from build123d import *

# Parameters (mm, degrees)
SCHIZZO1_W                   = 25
SCHIZZO1_H                   = 2
ESTRUSIONE_ESTRUSIONE1_DEPTH = 47
SCHIZZO2_W                   = 25
SCHIZZO2_H                   = 2
ESTRUSIONE_ESTRUSIONE2_DEPTH = 6
FORO_FILETTATO_M3X0_5_1_D    = 2.5
RACCORDO1_R                  = 5
ESTRUSIONE_ESTRUSIONE3_DEPTH = 4


with BuildPart() as part:
    # Schizzo1 → Estrusione-Estrusione1 (new body)
    with BuildSketch(Plane.XY):
        with Locations((-25, 9)):
            Rectangle(SCHIZZO1_W, SCHIZZO1_H)
    extrude(amount=-ESTRUSIONE_ESTRUSIONE1_DEPTH)

    # Schizzo2 → Estrusione-Estrusione2 (add)
    with BuildSketch(Plane.XY):
        with Locations((-25, 9)):
            Rectangle(SCHIZZO2_W, SCHIZZO2_H)
    extrude(amount=ESTRUSIONE_ESTRUSIONE2_DEPTH)

    # Foro filettato M3x0.5-1 (through all)
    with Locations(Plane(origin=(0, 10, 0), x_dir=(1, 0, 0), z_dir=(0, 1, 0))):
        with Locations((-25, -3)):
            Hole(FORO_FILETTATO_M3X0_5_1_D / 2)

    # Raccordo1
    raccordo1_edges = [part.edges().sort_by_distance(p)[0] for p in [
        (-37.5, 9, 6),
        (-12.5, 9, 6),
    ]]
    fillet(raccordo1_edges, radius=RACCORDO1_R)

    # Schizzo5 → Estrusione-Estrusione3 (add)
    with BuildSketch(Plane(origin=(0, 0, -47), x_dir=(-1, 0, 0), z_dir=(0, 0, -1))):
        Polygon((12.5, 10), (12.5, 12), (37.5, 12), (37.5, 10), (37.5, 8), (12.5, 8), align=None)
    extrude(amount=ESTRUSIONE_ESTRUSIONE3_DEPTH)


solid = part.part
Design review of the part built by this model. Coordinates are the model's own, in mm. A direction names the side the tool comes from. Coordinates: 2 decimals unless noted, no trailing zeros. Write each loop counter-clockwise with the first axis right and the second up, starting at its lowest first coordinate (ties: lowest second). Pieces come first, ordered by that corner, then holes. Notation, with made-up numbers: (-26.75, 21.5) - (-17.75, 21.5) arc R9 ccw to (-17.75, 34.5) - close; hole circle Ø3 at (-32.5, -11). An arc over 180 degrees is marked (long way). Use one line per item in the form item = value.
Q1. The part is to be moulded in two halves that separate along Z. For faces 3 (the flat face through (-25, 10, -51)), 4 (the cylindrical face through (-26.155, 8.986, 3.479)), 5 (the flat face through (-25, 11, -47)), 6 (the flat face through (-12.5, 9, -25)), say which applies: +Z half, -Z half, draft (parallel to the pull), parting line (faces both ways), or undercut.
Taken from the geometry:
face_3 = -Z half
face_4 = undercut
face_5 = +Z half
face_6 = draft
Q2. Consider section D-D (y = 10.7). Write out the cut boundary in (x, z), plus the area to 3 significant figures.
Taken from the geometry:
outline = (-37.5, -51) - (-12.5, -51) - (-12.5, -47) - (-37.5, -47) - close
area = 100 mm^2
Q3. Insertion check: pin 1 Ø1.5 at (x, z) = (-25, 3) entering from +Y; pin 2 Ø1.5 at (x, z) = (-29.5, -41) entering from +Y; pin 3 Ø0.6 at (x, y) = (-22.5, 11) entering from +Z. Each pin has a flat end and moves straight along its axis. Give the tip position at first contact, or say it passes through.
Taken from the geometry:
pin_1 = through
pin_2 = 10
pin_3 = -47
Q4. Consider section C-C (x = -31). Write out the cut boundary in (y, z), plus the area to 3 significant figures.
Taken from the geometry:
outline = (8, -51) - (12, -51) - (12, -47) - (10, -47) - (10, 6) - (8, 6) - close
area = 122 mm^2
Q5. Machinability: for faces 1 (the flat face through (-25, 10, -21)), 2 (the flat face through (-25, 12, -49)), which of the approach directions +Z, -Z, +X, -X, +Y, -Y give a long, thin tool a straight path to every point of the face, cutting with its end or side? Answer none if there is none.
Taken from the geometry:
face_1 = +Z, +X, -X, +Y
face_2 = +Z, -Z, +X, -X, +Y
Q6. Consider section B-B (z = 3). Write out the cut boundary in (x, y).
Taken from the geometry:
outline = (-37.08, 8) - (-26.25, 8) - (-26.25, 10) - (-37.08, 10) - close; (-23.75, 8) - (-12.92, 8) - (-12.92, 10) - (-23.75, 10) - close
Q7. For probe 1 along Z at (x, y) = (-25, 9.35); probe 2 along Y at (x, z) = (-17, -35.5); probe 3 along Z at (x, y) = (-22.25, 10.65), list the stretches that pass through material, from the lowest coordinate up.
Taken from the geometry:
probe_1 = -51 to 1.75, 4.25 to 6
probe_2 = 8 to 10
probe_3 = -51 to -47
Q8. Consider section A-A (x = -25). Write out the cut boundary in (y, z), plus the area to 3 significant figures.
Taken from the geometry:
outline = (8, -51) - (12, -51) - (12, -47) - (10, -47) - (10, 1.75) - (8, 1.75) - close; (8, 4.25) - (10, 4.25) - (10, 6) - (8, 6) - close
area = 117 mm^2
